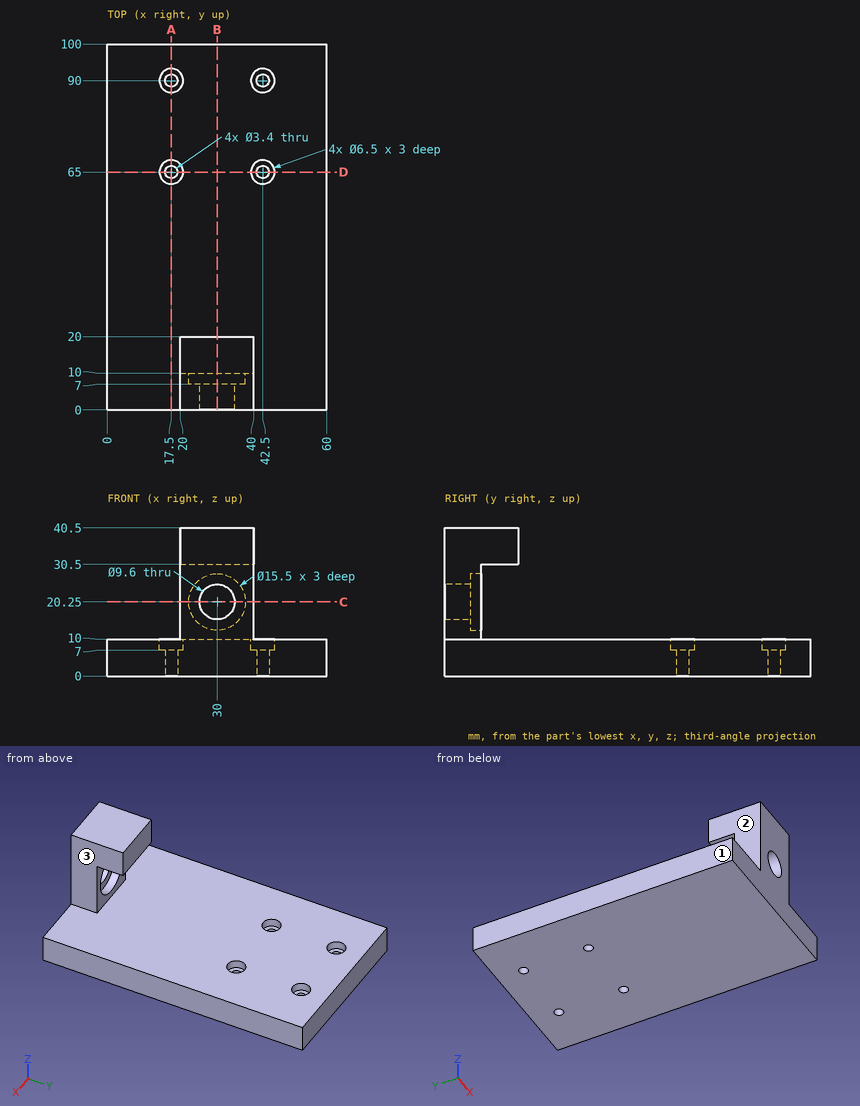
Answer from the drawing. Dimensions are ordinates in mm from the lowest x, y and z of the part. A direction names the side the tool comes from. Give positions to 0.01 mm unless a question says otherwise; leave off trailing zeros. Write each loop counter-clockwise with the first axis right and the second up, starting at its lowest first coordinate (ties: lowest second). Pieces come first, ordered by that corner, then holes. Notation, with made-up numbers: (-39.75, -16) -> (15.25, -16) arc R17 ccw to (15.25, -4) -> close; hole circle Ø3 at (38.25, -31). An arc over 180 degrees is marked (long way). One line per question, with ' | ' between items. Start each with the question number.
1. Section B-B (x = 30) is taken. Determine the outline of the cut face in (y, z).
2. Find the intervals of material crossed by probe 1 along Y at (x, z) = (42.5, 3.25); probe 2 along X at (y, z) = (90, 4.25); probe 3 along Y at (x, z) = (42, 4), in increasing order.
3. Section A-A (x = 17.5) is taken. Determine the outline of the cut face in (y, z).
4. For the marked faces 1, 2 and 3, determine the directions among +Z, -Z, +X, -X, +Y, -Y from which every point of the face is accessible in a straight line to the end or side of a thin tool.
5. Given pin 1 Ø7 at (x, y) = (17, 88.5) entering from +Z; pin 2 Ø2 at (x, y) = (43.5, 91.5) entering from +Z; pin 3 Ø6 at (x, z) = (29.5, 21.5) entering from +Y; pin 4 Ø12.5 at (x, z) = (28.5, 23.5) entering from +Y, each flat-ended and moving along its own axis, determine where each tip first touches the part or whether it passes through.
6. Section C-C (z = 20.25) is taken. Determine the outline of the cut face in (x, y), plus the area to 3 significant figures.
7. Section D-D (y = 65) is taken. Determine the outline of the cut face in (x, z).
Response values:
1) outline: (0, 0) -> (100, 0) -> (100, 10) -> (10, 10) -> (10, 12.5) -> (7, 12.5) -> (7, 15.45) -> (0, 15.45) -> close; (0, 25.05) -> (7, 25.05) -> (7, 28) -> (10, 28) -> (10, 30.5) -> (20, 30.5) -> (20, 40.5) -> (0, 40.5) -> close
2) probe 1: 0 to 63.3, 66.7 to 88.3, 91.7 to 100 | probe 2: 0 to 15.8, 19.2 to 40.8, 44.2 to 60 | probe 3: 0 to 63.38, 66.62 to 88.38, 91.62 to 100
3) outline: (0, 0) -> (63.3, 0) -> (63.3, 7) -> (61.75, 7) -> (61.75, 10) -> (0, 10) -> close; (66.7, 0) -> (88.3, 0) -> (88.3, 7) -> (86.75, 7) -> (86.75, 10) -> (68.25, 10) -> (68.25, 7) -> (66.7, 7) -> close; (91.7, 0) -> (100, 0) -> (100, 10) -> (93.25, 10) -> (93.25, 7) -> (91.7, 7) -> close
4) face 1: +Z, -Z, -X, +Y, -Y | face 2: +Z, -X, +Y, -Y | face 3: +Z, +X, +Y, -Y
5) pin 1: z = 10 | pin 2: z = 7 | pin 3: through | pin 4: y = 10
6) outline: (20, 0) -> (25.2, 0) -> (25.2, 7) -> (22.25, 7) -> (22.25, 10) -> (20, 10) -> close; (34.8, 0) -> (40, 0) -> (40, 10) -> (37.75, 10) -> (37.75, 7) -> (34.8, 7) -> close | area: 86.3 mm2
7) outline: (0, 0) -> (15.8, 0) -> (15.8, 7) -> (14.25, 7) -> (14.25, 10) -> (0, 10) -> close; (19.2, 0) -> (40.8, 0) -> (40.8, 7) -> (39.25, 7) -> (39.25, 10) -> (20.75, 10) -> (20.75, 7) -> (19.2, 7) -> close; (44.2, 0) -> (60, 0) -> (60, 10) -> (45.75, 10) -> (45.75, 7) -> (44.2, 7) -> close
